from build123d import *

# Parameters (mm, degrees)
F1_DEPTH     = 6.35
F2_SIZE      = 5.08
F4_DEPTH     = 3.175
F5_SIZE      = 3.17499
F6_R         = 0.635
F7_R         = 1.5875
F7_R_2       = 6.0325
F7_R_3       = 4.7625
F8_DEPTH     = 3.175
F8_TAPER     = 5
F9_T6_ANGLE  = 356.192567219
F9_T8_ANGLE  = 356.192567219
F9_T10_ANGLE = 238.0962831022
F9_T12_ANGLE = 118.0119864136
F9_T14_ANGLE = 178.0330528129
F9_T16_ANGLE = 178.0330528129
F9_T18_ANGLE = 118.0119864072
F9_T20_ANGLE = 238.0962831022
F9_T22_ANGLE = 356.192567219


# Not quite as in the source:
# - a fillet or chamfer that OpenCascade refuses, or shapes differently, is made with other operations: its cross-section is extruded or revolved along the edge and cut away or added
# - a fillet or chamfer is up to 0.001 mm smaller than in the source, because OpenCascade refuses the exact size


with BuildPart() as f1:
    # F0 (on Front) → F1 (new body)
    with BuildSketch(Plane.XZ):
        Polygon((-12.7, 21.9970452561), (-25.4, 0), (-12.7, -21.9970452561), (12.7, -21.9970452561), (25.4, 0), (12.7, 21.9970452561), align=None)
    extrude(amount=F1_DEPTH)

    # F2
    f2_edges = [f1.edges().sort_by_distance(p)[0] for p in [
        (0, -6.35, -21.997045),
        (19.05, -6.35, -10.998523),
        (19.05, -6.35, 10.998523),
        (0, -6.35, 21.997045),
        (-19.05, -6.35, 10.998523),
        (-19.05, -6.35, -10.998523),
    ]]
    chamfer(f2_edges, length=F2_SIZE)

    # F3 (on face) → F4 (cut)
    with BuildSketch(Plane.XZ.offset(6.35)):
        Polygon((7.9339735278, 13.7420452561), (-7.9339735278, 13.7420452561), (-15.8679470557, 0), (-7.9339735278, -13.7420452561), (7.9339735278, -13.7420452561), (15.8679470557, 0), align=None)
    extrude(amount=-F4_DEPTH, mode=Mode.SUBTRACT)

    # F5 (size 3.175 in the source; OpenCascade refuses exactly that, so slightly less here)
    f5_edges = [f1.edges().sort_by_distance(p)[0] for p in [
        (-11.90096, -3.175, 6.871023),
        (0, -3.175, 13.742045),
        (-11.90096, -3.175, -6.871023),
        (0, -3.175, -13.742045),
        (11.90096, -3.175, -6.871023),
        (11.90096, -3.175, 6.871023),
    ]]
    chamfer(f5_edges, length=F5_SIZE)

    # F6
    f6_edges = [f1.edges().sort_by_distance(p)[0] for p in [
        (19.05, 0, -10.998523),
        (19.05, 0, 10.998523),
        (0, 0, -21.997045),
        (-19.05, 0, -10.998523),
        (-19.05, 0, 10.998523),
        (0, 0, 21.997045),
    ]]
    fillet(f6_edges, radius=F6_R)

    # F7 (on face) → F8 (join)
    with BuildSketch(Plane.XZ.offset(3.175)):
        with Locations((12.2017728463, 0)):
            Circle(F7_R)
        Circle(F7_R_2)
        Circle(F7_R_3, mode=Mode.SUBTRACT)
        with Locations((6.1008864232, 10.5670452561)):
            Circle(F7_R)
        with Locations((-6.1008864232, 10.5670452561)):
            Circle(F7_R)
        with Locations((-12.2017728463, 0)):
            Circle(F7_R)
        with Locations((-6.1008864232, -10.5670452561)):
            Circle(F7_R)
        with Locations((6.1008864232, -10.5670452561)):
            Circle(F7_R)
    extrude(amount=F8_DEPTH, taper=F8_TAPER)

    # F9: chamfer of 1.27 on 11 edges, made by hand

    # F9_s1 → F9_t2 (revolve)
    with BuildSketch(Plane.XY):
        Polygon((4.8731877933, -4.4401672666), (3.4925, -3.175), (4.7625, -3.175), align=None)
    revolve(axis=Axis((0, -3.175, 0), (0, -1, 0)))

    # F9_s3 → F9_t4 (revolve)
    with BuildSketch(Plane.XY):
        Polygon((7.3025, -3.175), (5.9218122067, -4.4401672666), (6.0325, -3.175), align=None)
    revolve(axis=Axis((0, -3.175, 0), (0, -1, 0)))

    # F9_s5 → F9_t6 (revolve)
    with BuildSketch(Plane(origin=(0.0134654957, 0, -0.4051192424), x_dir=(0, 1, 0), z_dir=(0.0332200059, 0, -0.9994480633))):
        Polygon((-3.175, 15.0525382399), (-4.4401672666, 13.6718504466), (-3.175, 13.7825382399), align=None)
    revolve(axis=Axis((12.2017728463, -3.175, 0), (0, -1, 0)), revolution_arc=F9_T6_ANGLE)

    # F9_s7 → F9_t8 (revolve)
    with BuildSketch(Plane(origin=(0.3575763033, 0, -0.1908981598), x_dir=(0, 1, 0), z_dir=(0.8821574155, 0, -0.4709546626))):
        Polygon((-4.4401672666, 13.6718504466), (-3.175, 15.0525382399), (-3.175, 13.7825382399), align=None)
    revolve(axis=Axis((6.1008864232, -3.175, 10.5670452561), (0, -1, 0)), revolution_arc=F9_T8_ANGLE)

    # F9_s9 → F9_t10 (revolve)
    with BuildSketch(Plane(origin=(0.3441108974, 0, 0.2142211427), x_dir=(0, 1, 0), z_dir=(0.8489374049, 0, 0.5284934082))):
        Polygon((-3.175, 15.0525382363), (-4.4401672666, 13.671850443), (-3.175, 13.7825382363), align=None)
    revolve(axis=Axis((-6.1008864232, -3.175, 10.5670452561), (0, -1, 0)), revolution_arc=F9_T10_ANGLE)

    # F9_s11 → F9_t12 (revolve)
    with BuildSketch(Plane.XY.offset(10.5670452561)):
        Polygon((-3.2433864232, -3.175), (-4.6240742165, -4.4401672666), (-4.5133864232, -3.175), align=None)
    revolve(axis=Axis((-6.1008864232, -3.175, 10.5670452561), (0, -1, 0)), revolution_arc=F9_T12_ANGLE)

    # F9_s13 → F9_t14 (revolve)
    with BuildSketch(Plane(origin=(-0.0143744903, 0, 0.4185542247), x_dir=(0, 1, 0), z_dir=(-0.0343229619, 0, 0.9994107936))):
        Polygon((-3.175, 15.0520834832), (-4.4401672666, 13.6713956899), (-3.175, 13.7820834832), align=None)
    revolve(axis=Axis((-12.2017728463, -3.175, 0), (0, -1, 0)), revolution_arc=F9_T14_ANGLE)

    # F9_s15 → F9_t16 (revolve)
    with BuildSketch(Plane.XY):
        Polygon((-9.3442728463, -3.175), (-10.7249606396, -4.4401672666), (-10.6142728463, -3.175), align=None)
    revolve(axis=Axis((-12.2017728463, -3.175, 0), (0, -1, 0)), revolution_arc=F9_T16_ANGLE)

    # F9_s17 → F9_t18 (revolve)
    with BuildSketch(Plane(origin=(-0.3736965716, 0, 0.1987982832), x_dir=(0, 1, 0), z_dir=(-0.882849359, 0, 0.4696562672))):
        Polygon((-3.175, 15.0519286749), (-4.4401672666, 13.6712408817), (-3.175, 13.7819286749), align=None)
    revolve(axis=Axis((-6.1008864232, -3.175, -10.5670452561), (0, -1, 0)), revolution_arc=F9_T18_ANGLE)

    # F9_s19 → F9_t20 (revolve)
    with BuildSketch(Plane.XY.offset(-10.5670452561)):
        Polygon((-3.2433864232, -3.175), (-4.6240742165, -4.4401672666), (-4.5133864232, -3.175), align=None)
    revolve(axis=Axis((-6.1008864232, -3.175, -10.5670452561), (0, -1, 0)), revolution_arc=F9_T20_ANGLE)

    # F9_s21 → F9_t22 (revolve)
    with BuildSketch(Plane(origin=(-0.3441108076, 0, -0.2142210826), x_dir=(0, 1, 0), z_dir=(-0.8489374096, 0, -0.5284934007))):
        Polygon((-3.175, 15.0525382399), (-4.4401672666, 13.6718504466), (-3.175, 13.7825382399), align=None)
    revolve(axis=Axis((6.1008864232, -3.175, -10.5670452561), (0, -1, 0)), revolution_arc=F9_T22_ANGLE)


solid = f1.part
Part model, mm, in its own coordinate system. A direction names the side the tool comes from. Give positions to 0.01 mm unless a question says otherwise; leave off trailing zeros. Loops run counter-clockwise (first coordinate to the right, second up) from the corner with the lowest first, then second, coordinate; pieces in that order, holes last.
(1) 3-axis set-ups, long thin cutter, end or side, ignore diameter. For faces 1 (the flat face through (1, -6.35, 14)), 2 (the flat face through (0, -3.175, 0)): which of +Z, -Z, +X, -X, +Y, -Y reach the whole face in a straight line?
Return value:
face 1: +Z, -Z, +X, -X, -Y
face 2: -Y
(2) Band-saw the part on C-C (y = -2.5). Write the cut outline in (x, z).
Return value:
outline: (-23.98, 0) - (-11.99, -20.77) - (11.99, -20.77) - (23.98, 0) - (11.99, 20.77) - (-11.99, 20.77) - close
(3) Band-saw the part on A-A (y = -5.5). Count the separate pieces of the cut face and the enclosed holes in it, and give its area (3 significant figures).
Return value:
separate pieces: 8
enclosed holes: 2
area: 583 mm2
(4) Pin check, flat tips, straight feed: pin 1 (1 mm diameter, centred on y = -1, z = -17.5, fed in from +X); pin 2 (1 mm diameter, centred on x = -16.5, z = -15.5, fed in from -Y); pin 3 (3 mm diameter, centred on y = -3.5, z = -9.5, fed in from -X). Stop position of each tip, or through.
Return value:
pin 1: stops at x = 15.59
pin 2: stops at y = -1.73
pin 3: stops at x = -19.28
(5) Drill centre lines: line 1 along Y through (x, z) = (13, 1.5); line 2 along X through (y, z) = (-5.5, -0.5); line 3 along Y through (x, z) = (10, 2.5) (3 decimals). Where is each one in solid material? Low to high.
Return value:
line 1: y = -4.62 to 0
line 2: x = -20.23 to -14.6, -13.49 to -10.91, -5.81 to -4.94, 4.94 to 5.81, 10.91 to 13.49, 14.6 to 20.23
line 3: y = -3.175 to 0
(6) Pull direction X, two halves, no side cores. Call faces 3 (the conical face through (5.2, -4.22, 9.106)), 4 (the cylindrical face through (18.982, -0.191, -10.754)), 5 (the cylindrical face through (-18.982, -0.191, 10.754)): pulls with the +X half, pulls with the -X half, needs draft (parallel to the pull), parting line crosses it, or undercut.
Return value:
face 3: undercut
face 4: pulls with the +X half
face 5: pulls with the -X half
